Can you work these out from the model? Positions are in its coordinate system, mm. Face numbers are marked on the shaded views. Round coordinates to 2 decimals unless told otherwise and drop trailing zeros. Write each loop counter-clockwise with the first axis right and the second up, starting at its lowest first coordinate (ties: lowest second). Pieces come first, ordered by that corner, then holes. Notation, with made-up numbers: (47, -3.5) -> (79, -3.5) arc R28 ccw to (79, 19.5) -> close; hole circle Ø7 at (61.5, -25). An arc over 180 degrees is marked (long way). Write item = value, one per line. Start each with the question number.
1) If I drill on line 1 (X direction, y = -0.9, z = -15.5); line 2 (X direction, y = 2.4, z = 15.5); line 3 (Z direction, x = -15.5, y = 2.45), over which ranges is the centre line in solid material (lowest first)?
2) Thinking about a two-plate mould opening in X: for the marked faces 1, 2 and 3, which applies, +X half, -X half, draft (parallel to the pull), parting line (faces both ways), or undercut?
3) Imagine slicing it at D-D, the plane x = -15.5. Please give me the cut outline in (y, z) (3 decimals).
4) Imagine slicing it at A-A, the plane x = 0. Please give me the cut outline in (y, z), then the cut area to 4 significant figures.
5) Imagine slicing it at C-C, the plane z = 2. Please give me the cut outline in (x, y).
6) Imagine slicing it at B-B, the plane y = -0.8. Please give me the cut outline in (x, z), then the cut area to 3 significant figures.
from build123d import *

# Parameters (mm, degrees)
ESBO_O1_W                                    = 45
ESBO_O1_H                                    = 45
ESBO_O1_R                                    = 9.75
RESSALTO_EXTRUS_O1_DEPTH                     = 2.5
ESCAREADO_PARA_PARAFUSO_COM_CABE_A_E_2_COUNT = 2
ESCAREADO_PARA_PARAFUSO_COM_CABE_A_E_2_PITCH = 31
ESCAREADO_PARA_PARAFUSO_COM_CABE_A_E_3_COUNT = 2
ESCAREADO_PARA_PARAFUSO_COM_CABE_A_E_3_PITCH = 43.840620434
ESCAREADO_PARA_PARAFUSO_COM_CABE_A_E_4_COUNT = 2
ESCAREADO_PARA_PARAFUSO_COM_CABE_A_E_4_PITCH = 31
FILETE1_R                                    = 5


with BuildPart() as part:
    # Esboço1 → Ressalto-extrusão1 (new, symmetric)
    with BuildSketch(Plane(origin=(0, 0, 0), x_dir=(1, 0, 0), z_dir=(0, 1, 0))):
        Rectangle(ESBO_O1_W, ESBO_O1_H)
        with Locations(Location((0, 0, 0), (0, 0, 270))):
            Circle(ESBO_O1_R, mode=Mode.SUBTRACT)
    extrude(amount=RESSALTO_EXTRUS_O1_DEPTH, both=True)

    # Esboço4 → Escareado para parafuso com cabeça escareada elevada de M31 (revolve, cut)
    with BuildSketch(Plane(origin=(-15.5, 2.5, -15.5), x_dir=(0, 0, 1), z_dir=(1, 0, 0))):
        Polygon((0, 0), (0, 5), (1.725, 5), (1.7, 4.975), (1.7, 1.65), (3.15, 0.2), (3.15, 0), align=None)
    escareado_para_parafuso_com_cabe_a_escar = revolve(axis=Axis((-15.5, 8.85, -15.5), (0, -1, 0)), mode=Mode.SUBTRACT)

    # Escareado para parafuso com cabe_a e 2: Escareado para parafuso com cabeça escareada elevada de M31 ×2
    with Locations(*[(i * ESCAREADO_PARA_PARAFUSO_COM_CABE_A_E_2_PITCH, 0, 0) for i in range(1, ESCAREADO_PARA_PARAFUSO_COM_CABE_A_E_2_COUNT)]):
        add(escareado_para_parafuso_com_cabe_a_escar, mode=Mode.SUBTRACT)

    # Escareado para parafuso com cabe_a e 3: Escareado para parafuso com cabeça escareada elevada de M31 ×2
    with Locations(*[Vector(0.7071067811865447, 0, 0.7071067811865503) * (i * ESCAREADO_PARA_PARAFUSO_COM_CABE_A_E_3_PITCH) for i in range(1, ESCAREADO_PARA_PARAFUSO_COM_CABE_A_E_3_COUNT)]):
        add(escareado_para_parafuso_com_cabe_a_escar, mode=Mode.SUBTRACT)

    # Escareado para parafuso com cabe_a e 4: Escareado para parafuso com cabeça escareada elevada de M31 ×2
    with Locations(*[(0, 0, i * ESCAREADO_PARA_PARAFUSO_COM_CABE_A_E_4_PITCH) for i in range(1, ESCAREADO_PARA_PARAFUSO_COM_CABE_A_E_4_COUNT)]):
        add(escareado_para_parafuso_com_cabe_a_escar, mode=Mode.SUBTRACT)

    # Filete1
    filete1_edges = [part.edges().sort_by_distance(p)[0] for p in [
        (22.5, 0, 22.5),
        (-22.5, 0, 22.5),
        (-22.5, 0, -22.5),
        (22.5, 0, -22.5),
    ]]
    fillet(filete1_edges, radius=FILETE1_R)

    # Esboço5 → Furo de diâmetro Ø5.2 (5.2)1 (revolve, cut)
    with BuildSketch(Plane(origin=(17.5, -2.5, 0), x_dir=(0, 0, -1), z_dir=(1, 0, 0))):
        Polygon((0, 0), (0, 47.562237609), (2.6, 46), (2.6, 0), align=None)
    furo_de_di_metro_5_2_5_2_1 = revolve(axis=Axis((17.5, -8.85, 0), (0, 1, 0)), mode=Mode.SUBTRACT)

    # Espelhar1: Furo de diâmetro Ø5.2 (5.2)1 across plane
    add(furo_de_di_metro_5_2_5_2_1.mirror(Plane(origin=(0, 0, 0), x_dir=(0, 0, 1), z_dir=(1, 0, 0))), mode=Mode.SUBTRACT)


solid = part.part
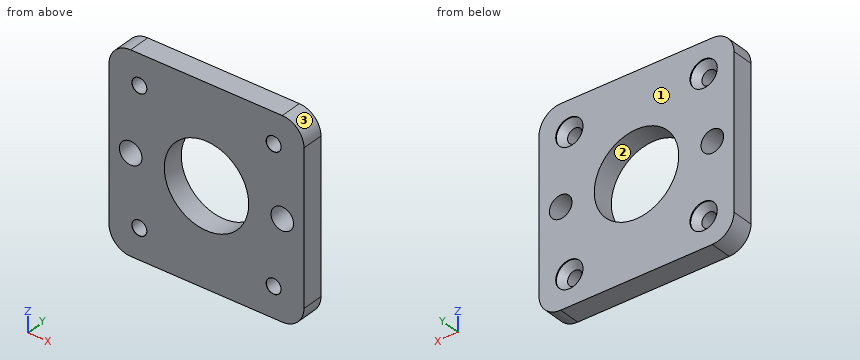
Reported:
q1.line_1 = -22.5 to -17.2, -13.8 to 13.8, 17.2 to 22.5
q1.line_2 = -22.5 to -18.65, -12.35 to 12.35, 18.65 to 22.5
q1.line_3 = -22.5 to -18.65, -12.35 to -1.66, 1.66 to 12.35, 18.65 to 22.5
q2.face_1 = draft
q2.face_2 = undercut
q2.face_3 = +X half
q3.outline = (-2.5, -22.5) -> (2.5, -22.5) -> (2.5, -18.65) -> (2.3, -18.65) -> (0.85, -17.2) -> (-2.475, -17.2) -> (-2.5, -17.225) -> close; (-2.5, -13.775) -> (-2.475, -13.8) -> (0.85, -13.8) -> (2.3, -12.35) -> (2.5, -12.35) -> (2.5, -1.661) -> (-2.5, -1.661) -> close; (-2.5, 1.661) -> (2.5, 1.661) -> (2.5, 12.35) -> (2.3, 12.35) -> (0.85, 13.8) -> (-2.475, 13.8) -> (-2.5, 13.775) -> close; (-2.5, 17.225) -> (-2.475, 17.2) -> (0.85, 17.2) -> (2.3, 18.65) -> (2.5, 18.65) -> (2.5, 22.5) -> (-2.5, 22.5) -> close
q4.outline = (-2.5, -22.5) -> (2.5, -22.5) -> (2.5, -9.75) -> (-2.5, -9.75) -> close; (-2.5, 9.75) -> (2.5, 9.75) -> (2.5, 22.5) -> (-2.5, 22.5) -> close
q4.area = 127.5 mm²
q5.outline = (-22.5, -2.5) -> (-19.16, -2.5) -> (-19.16, 2.5) -> (-22.5, 2.5) -> close; (-15.84, -2.5) -> (-9.54, -2.5) -> (-9.54, 2.5) -> (-15.84, 2.5) -> close; (9.54, -2.5) -> (15.84, -2.5) -> (15.84, 2.5) -> (9.54, 2.5) -> close; (19.16, -2.5) -> (22.5, -2.5) -> (22.5, 2.5) -> (19.16, 2.5) -> close
q6.outline = (-22.5, -17.5) arc R5 ccw to (-17.5, -22.5) -> (17.5, -22.5) arc R5 ccw to (22.5, -17.5) -> (22.5, 17.5) arc R5 ccw to (17.5, 22.5) -> (-17.5, 22.5) arc R5 ccw to (-22.5, 17.5) -> close; hole circle Ø5.2 at (-17.5, 0); hole circle Ø3.4 at (-15.5, -15.5); hole circle Ø3.4 at (-15.5, 15.5); hole circle Ø19.5 at (0, 0); hole circle Ø3.4 at (15.5, -15.5); hole circle Ø3.4 at (15.5, 15.5); hole circle Ø5.2 at (17.5, 0)
q6.area = 1,630 mm²
